from build123d import *

# Parameters (mm, degrees)
F0_R     = 15.7692613996
F1_DEPTH = 25
F2_R     = 2
F3_R     = 6.8344152612
F4_DEPTH = 40


# Not quite as in the source:
# - a feature names something its author has since deleted; it is built from what else it names


with BuildPart() as f1:
    # F0 (on Top) → F1 (new body)
    with BuildSketch(Plane.XY):
        with Locations((-22.6599406451, -18.1141793728)):
            Circle(F0_R)
    extrude(amount=F1_DEPTH)

    # F2
    f2_edges = [f1.edges().sort_by_distance(p)[0] for p in [
        (-38.429202, -18.114179, 0),
        (-38.429202, -18.114179, 25),
    ]]
    fillet(f2_edges, radius=F2_R)

    # F3 (on face) → F4 (cut)
    with BuildSketch(Plane(origin=(0, 0, 0), x_dir=(1, 0, 0), z_dir=(0, 0, -1))):
        with Locations((-22.6599406451, 18.1141793728)):
            Circle(F3_R)
    extrude(amount=-F4_DEPTH, mode=Mode.SUBTRACT)


solid = f1.part
Can you work these out from the model? Positions are in its coordinate system, mm. Coordinates: 2 decimals unless noted, no trailing zeros. Write each loop counter-clockwise with the first axis right and the second up, starting at its lowest first coordinate (ties: lowest second). Pieces come first, ordered by that corner, then holes. Notation, with made-up numbers: (24.25, 57.5) -> (28.25, 57.5) arc R15 ccw to (28.25, 78.5) -> close; hole circle Ø2 at (20, 3.25). An arc over 180 degrees is marked (long way). Write each question's results on one line, items separated by ' | '. Start each with the question number.
Q1. We'd pull the mould along Y, two halves only. Please class faces 1 (the face through (-16.14, -20.17, 12.32)), 2 (the face through (-15.383, -32.104, 12.353)), 3 (the face through (-29, -15, 0)): +Y half, -Y half, draft (parallel to the pull), parting line (faces both ways), or undercut.
Q2. I'm going to push flat-ended pins straight in: pin 1 (8 mm diameter, centred on x = -22.66, y = -18.11, fed in from +Z); pin 2 (10 mm diameter, centred on y = -30, z = 13.5, fed in from +X); pin 3 (4 mm diameter, centred on y = -12.5, z = 18, fed in from +X); pin 4 (10 mm diameter, centred on x = -34.5, z = 16, fed in from +Y). Where does each tip first touch, or does it pass through?
Q3. If I drill on probe 1 along X at (y, z) = (-18.5, 15.75); probe 2 along Y at (x, z) = (-16.5, 1.5); probe 3 along X at (y, z) = (-20, 15.25), over which ranges is the centre line in solid material (lowest first)?
Q4. Imagine slicing it at A-A (z = 23.75). Write out the boundary of the cut face in (x, y).
Q5. Imagine slicing it at B-B (z = 20.25). Write out the boundary of the cut face in (x, y).
Taken from the geometry:
1) face 1: undercut | face 2: parting line | face 3: draft
2) pin 1: passes through | pin 2: stops at x = -8.47 | pin 3: stops at x = -7.31 | pin 4: stops at y = -3.91
3) probe 1: x = -38.42 to -29.48, -15.84 to -6.9 | probe 2: y = -32.56 to -21.07, -15.15 to -3.67 | probe 3: x = -38.32 to -29.23, -16.09 to -7
4) outline: circle Ø31.25 at (-22.66, -18.11); hole circle Ø13.67 at (-22.66, -18.11)
5) outline: circle Ø31.54 at (-22.66, -18.11); hole circle Ø13.67 at (-22.66, -18.11)
